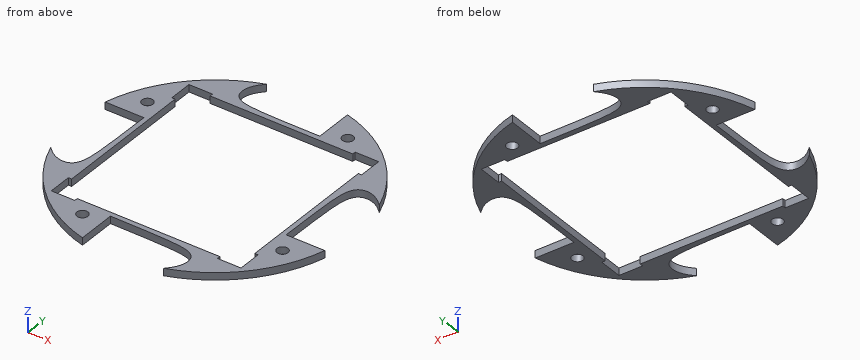
from build123d import *

# Parameters (mm, degrees)
BOSS_EXTRUDE3_OUTLINE_R = 3
BOSS_EXTRUDE3_DEPTH     = 4
CUT_EXTRUDE1_DEPTH      = 4
CUT_EXTRUDE2_DEPTH      = 4
SKETCH4_W               = 0.4
SKETCH4_H               = 1.8
SKETCH4_W_2             = 1.8
SKETCH4_H_2             = 0.4
BOSS_EXTRUDE4_DEPTH     = 4


# Read off the part's stored shape, not the designer's step: Boss-Extrude3
with BuildPart() as part:
    # Boss-Extrude3 outline → Boss-Extrude3 (new body)
    with BuildSketch(Plane.XY):
        with BuildLine():
            add(Edge.make_bspline(
                [(24.392810524, -72.348554199), (27.040667073, -69.541086329), (29.089162938, -67.428574969), (30.241441862, -64.355831171), (31.073643307, -60.963009895), (30.561519341, -59.042545022), (29.217193929, -56.673971678), (27.488775543, -54.241382838), (25.105954954, -53), (17.37432721, -53), (-19, -52.782560411)],
                knots=[0, 0, 0, 0, 0, 0, 0, 0, 0, 0, 0, 1, 1, 1, 1, 1, 1, 1, 1, 1, 1, 1], degree=10))
            ThreePointArc((24.392810524, -72.348554199), (55.939709188, -51.962211615), (73.948106805, -19))
            Line((73.948106805, -19), (52.782560411, -19))
            add(Edge.make_bspline(
                [(72.348554199, 24.392810524), (69.541086329, 27.040667073), (67.428574969, 29.089162938), (64.355831171, 30.241441862), (60.963009895, 31.073643307), (59.042545022, 30.561519341), (56.673971678, 29.217193929), (54.241382838, 27.488775543), (53, 25.105954954), (53, 17.37432721), (52.782560411, -19)],
                knots=[0, 0, 0, 0, 0, 0, 0, 0, 0, 0, 0, 1, 1, 1, 1, 1, 1, 1, 1, 1, 1, 1], degree=10))
            ThreePointArc((72.348554199, 24.392810524), (51.962211615, 55.939709188), (19, 73.948106805))
            Line((19, 73.948106805), (19, 53))
            add(Edge.make_bspline(
                [(-24.392810524, 72.348554199), (-27.040667073, 69.541086329), (-29.089162938, 67.428574969), (-30.241441862, 64.355831171), (-31.073643307, 60.963009895), (-30.561519341, 59.042545022), (-29.217193929, 56.673971678), (-27.488775543, 54.241382838), (-25.105954954, 53), (-17.37432721, 53), (19, 53)],
                knots=[0, 0, 0, 0, 0, 0, 0, 0, 0, 0, 0, 1, 1, 1, 1, 1, 1, 1, 1, 1, 1, 1], degree=10))
            ThreePointArc((-24.392810524, 72.348554199), (-55.939709188, 51.962211615), (-73.948106805, 19))
            Line((-73.948106805, 19), (-52.782560411, 19))
            add(Edge.make_bspline(
                [(-72.348554199, -24.392810524), (-69.541086329, -27.040667073), (-67.428574969, -29.089162938), (-64.355831171, -30.241441862), (-60.963009895, -31.073643307), (-59.042545022, -30.561519341), (-56.673971678, -29.217193929), (-54.241382838, -27.488775543), (-53, -25.105954954), (-53, -17.37432721), (-52.782560411, 19)],
                knots=[0, 0, 0, 0, 0, 0, 0, 0, 0, 0, 0, 1, 1, 1, 1, 1, 1, 1, 1, 1, 1, 1], degree=10))
            ThreePointArc((-72.348554199, -24.392810524), (-51.962211615, -55.939709188), (-19, -73.948106805))
            Line((-19, -73.948106805), (-19, -52.782560411))
        make_face()
        with Locations((-30, -58.782560411)):
            Circle(BOSS_EXTRUDE3_OUTLINE_R, mode=Mode.SUBTRACT)
        with Locations((58.782560411, -30)):
            Circle(BOSS_EXTRUDE3_OUTLINE_R, mode=Mode.SUBTRACT)
        with Locations((-58.782560411, 30)):
            Circle(BOSS_EXTRUDE3_OUTLINE_R, mode=Mode.SUBTRACT)
        Polygon((-38.9, -51.6), (-51.6, -51.6), (-51.6, -38.9), (-50, -38.9), (-50, 38.9), (-51.6, 38.9), (-51.6, 51.6), (-38.9, 51.6), (-38.9, 50), (38.9, 50), (38.9, 51.6), (51.6, 51.6), (51.6, 38.9), (50, 38.9), (50, -38.9), (51.6, -38.9), (51.6, -51.6), (38.9, -51.6), (38.9, -50), (-38.9, -50), align=None, mode=Mode.SUBTRACT)
        with Locations((30, 59)):
            Circle(BOSS_EXTRUDE3_OUTLINE_R, mode=Mode.SUBTRACT)
    extrude(amount=BOSS_EXTRUDE3_DEPTH)

    # Sketch2 → Cut-Extrude1 (cut)
    with BuildSketch(Plane.XY.offset(4)):
        Polygon((51.8, -38.7), (50.2, -38.7), (50.2, 38.7), (51.8, 38.7), (51.8, 51.8), (38.7, 51.8), (38.7, 50.2), (-38.7, 50.2), (-38.7, 51.8), (-51.8, 51.8), (-51.8, 38.7), (-50.2, 38.7), (-50.2, -38.7), (-51.8, -38.7), (-51.8, -51.8), (-38.7, -51.8), (-38.7, -50.2), (38.7, -50.2), (38.7, -51.8), (51.8, -51.8), align=None)
        Polygon((51.6, -38.9), (50, -38.9), (50, 38.9), (51.6, 38.9), (51.6, 51.6), (38.9, 51.6), (38.9, 50), (-38.9, 50), (-38.9, 51.6), (-51.6, 51.6), (-51.6, 38.9), (-50, 38.9), (-50, -38.9), (-51.6, -38.9), (-51.6, -51.6), (-38.9, -51.6), (-38.9, -50), (38.9, -50), (38.9, -51.6), (51.6, -51.6), align=None, mode=Mode.SUBTRACT)
    extrude(amount=-CUT_EXTRUDE1_DEPTH, mode=Mode.SUBTRACT)

    # Sketch3 → Cut-Extrude2 (cut)
    with BuildSketch(Plane.XY.offset(4)):
        Polygon((-51.8, -51.8), (-38.7, -51.8), (-38.7, -52), (-52, -52), (-52, -38.7), (-51.8, -38.7), align=None)
        Polygon((38.7, -51.8), (51.8, -51.8), (51.8, -38.7), (52, -38.7), (52, -52), (38.7, -52), align=None)
        Polygon((51.8, 38.7), (51.8, 51.8), (38.7, 51.8), (38.7, 52), (52, 52), (52, 38.7), align=None)
        Polygon((-51.8, 51.8), (-51.8, 38.7), (-52, 38.7), (-52, 52), (-38.7, 52), (-38.7, 51.8), align=None)
    extrude(amount=-CUT_EXTRUDE2_DEPTH, mode=Mode.SUBTRACT)

    # Sketch4 → Boss-Extrude4 (add)
    with BuildSketch(Plane.XY.offset(4)):
        with Locations((-38.9, 51.1)):
            Rectangle(SKETCH4_W, SKETCH4_H)
        with Locations((-51.1, 38.9)):
            Rectangle(SKETCH4_W_2, SKETCH4_H_2)
        with Locations((38.9, 51.1)):
            Rectangle(SKETCH4_W, SKETCH4_H)
        with Locations((51.1, 38.9)):
            Rectangle(SKETCH4_W_2, SKETCH4_H_2)
        with Locations((38.9, -51.1)):
            Rectangle(SKETCH4_W, SKETCH4_H)
        with Locations((51.1, -38.9)):
            Rectangle(SKETCH4_W_2, SKETCH4_H_2)
        with Locations((-51.1, -38.9)):
            Rectangle(SKETCH4_W_2, SKETCH4_H_2)
        with Locations((-38.9, -51.1)):
            Rectangle(SKETCH4_W, SKETCH4_H)
    extrude(amount=-BOSS_EXTRUDE4_DEPTH)


solid = part.part
The listing builds one solid part. Answer for the finished solid, in the listing's coordinates (mm). Round coordinates to 2 decimals unless told otherwise and drop trailing zeros. Use one line per item in the form item = value. Start each with the question number.
Item 1: A cutting plane is placed at A-A (x = 58). Give the number of separate pieces and of enclosed holes in the cut face, plus the area to 3 significant figures.
Item 2: Flat-ended cylindrical pins translate along their axes: pin 1 Ø2 at (y, z) = (-45, 1) entering from -X; pin 2 Ø1 at (x, z) = (12, 1.5) entering from +Y; pin 3 Ø2 at (y, z) = (51, 2) entering from +X; pin 4 Ø8 at (x, y) = (-58.78, 30) entering from +Z. Find the tip coordinate at first contact, or state that the pin passes through.
Item 3: Find the intervals of material crossed by line 1 (X direction, y = 32, z = 2.25); line 2 (Y direction, x = 30, z = 1.95); line 3 (Y direction, x = -31, z = 3.3), in increasing order. Write a range as [from, to].
The answers:
q1.separate_pieces = 3
q1.enclosed_holes = 0
q1.area = 182 mm^2
q2.pin_1 = -62.4
q2.pin_2 = 53
q2.pin_3 = 57.7
q2.pin_4 = 4
q3.line_1 = [-69.32, -61.02], [-56.55, -50.2], [50.2, 69.32]
q3.line_2 = [-70.21, -50.2], [50.2, 56], [62, 70.21]
q3.line_3 = [-69.77, -61.61], [-55.95, -50.2], [50.2, 69.77]
